Autodesk Inventor part; units mm, degrees
ref_plane "YZ Plane" through (0, 0, 0) normal (1, 0, 0) x (0, 1, 0)
ref_plane "XZ Plane" through (0, 0, 0) normal (0, 1, 0) x (-1, 0, 0)
ref_plane "XY Plane" through (0, 0, 0) normal (0, 0, 1) x (1, 0, 0)
sketch "Sketch1" plane through (0, 0, 0) normal (0, 0, 1) x (1, 0, 0)
  line L0 (0, 0) -> (88.9, 0)
  line L1 (88.9, 0) -> (88.9, 12.7)
  line L2 (0, 12.7) -> (0, 0)
  line L3 (0, 12.7) -> (0, 0)
  circle A0 centre (37.338, 50.8) radius 14.2875
  line L4 (0, 0) -> (0, 12.7)
  line L5 (0, 0) -> (0, 12.7)
  line L6 (0, 12.7) -> (15.748, 12.7)
  line L7 (13.208, 0) -> (0, 0)
  line L8 (15.748, 12.7) -> (0, 12.7)
  line L9 (15.748, 54.61) -> (15.748, 12.7)
  line L10 (88.9, 0) -> (62.992, 0)
  line L11 (73.152, 12.7) -> (88.9, 12.7)
  line L12 (88.9, 12.7) -> (88.9, 0)
  line L13 (73.152, 12.7) -> (73.152, 54.61)
  line L14 (60.452, 71.222) -> (28.448, 71.222)
  line L15 (15.748, 54.61) -> (15.748, 58.522)
  line L16 (73.152, 58.522) -> (73.152, 54.61)
  arc A1 (28.448, 71.222) -> (15.748, 58.522) centre (28.448, 58.522) ccw
  arc A2 (73.152, 58.522) -> (60.452, 71.222) centre (60.452, 58.522) ccw
  point P0 (65.9232, 76.2)
  point P1 (0, 12.7)
  dimension "d9" = 28.575
  dimension "d10" = 88.9
  dimension "d56" = 12.7
  dimension "d57" = 15.748
  dimension "d79" = 21.59
  dimension "d83" = 15.748
  dimension "d87" = 12.7
  dimension "d111" = 41.91
  dimension "d112" = 41.91
  dimension "d118" = 25.4
  dimension "d119" = 12.7
extrude "Extrusion7" add sketch "Sketch1" along normal blind 15.24
sketch "Sketch9" plane through (73.152, 12.7, 0) normal (0, 1, 0) x (1, 0, 0)
  point P0 (-73.152, 0)
  point P1 (8.0463, -7.7031)
hole "Hole4" at (81.1983, 12.7, 7.7031) direction (0, -1, 0) diameter 6.4008 end through all counterbore diameter 11.9062 counterbore depth 7.9502
sketch "Sketch10" plane through (0.0713, 12.7, -0.0767) normal (0, 1, 0) x (1, 0, 0)
  point P0 (-75.692, 0)
  point P1 (7.4278, -7.7745)
hole "Hole5" at (7.4991, 12.7, 7.6977) direction (0, -1, 0) diameter 6.4008 end through all counterbore diameter 11.9062 counterbore depth 7.9502
properties part number "Updated Support_chris"
The listing builds one solid part. Answer for the finished solid, in the listing's coordinates (mm). A direction names the side the tool comes from. Give positions to 0.01 mm unless a question says otherwise; leave off trailing zeros. Order: outer loops, then holes, each group sorted by start corner. A loop starts at its lowest first (then second) coordinate and runs counter-clockwise, first axis right, second up. Notation, with made-up numbers: M 61.25,-12 L 119.25,-12 A20 cw 119.25,17 Z; hole C -11.75,-9 d7. An arc over 180 degrees is marked long. Put each result on its own line as item: value. Start each with the question number.
Item 1: The part is cut by section C-C, the plane x = 12. Determine the outline of the cut face in (y, z), and give its area (3 significant figures).
Item 2: For a pull along Z with two mould halves and no side action, classify faces 1 (the face through (44, 28, 15.24)), 2 (the face through (45, 71.222, 8)), 3 (the face through (80.237, 2.342, 10.756)), 4 (the face through (4.326, 2.342, 7.281)) as +Z half, -Z half, draft (parallel to the pull), parting line (faces both ways), or undercut.
Item 3: The part is cut by section D-D, the plane y = 15.5. Determine the outline of the cut face in (x, z), and give its area (3 significant figures).
Item 4: Flat-ended cylindrical pins translate along their axes: P1, Ø1, axis at x = 67.5, z = 3.5, coming from the -Y side; P2, Ø17, axis at x = 37.338, y = 50.8, coming from the -Z side (3 decimals); P3, Ø2, axis at y = 60, z = 9.5, coming from the -X side; P4, Ø1, axis at y = 36.5, z = 2, coming from the -X side. Find the tip coordinate at first contact, or state that the pin passes through.
Item 5: The part is cut by section B-B, the plane y = 50.8. Determine the outline of the cut face in (x, z), and give its area (3 significant figures).
Item 6: The part is cut by section A-A, the plane z = 8. Determine the outline of the cut face in (x, y) (1 decimal), and give its area (3 significant figures).
Item 7: Find the intervals of material crossed by line 1 along X through (y, z) = (16, 7.75); line 2 along X through (y, z) = (48.5, 7.5); line 3 along Y through (x, z) = (76, 1.25), in increasing order.
Item 8: Which of the six approach directions +Z, -Z, +X, -X, +Y, -Y give full straight-line access (tool end or side, diameter ignored) to faces 5 (the face through (77, 12.7, 2)), 6 (the face through (10, 4.75, 10)), 7 (the face through (15.748, 36, 8))?
Answer key:
1. outline: M 0,0 L 12.7,0 L 12.7,3.8 L 4.75,3.8 L 4.75,11.59 L 12.7,11.59 L 12.7,15.24 L 0,15.24 Z
1. area: 132 mm²
2. face 1: +Z half
2. face 2: draft
2. face 3: undercut
2. face 4: undercut
3. outline: M 15.75,0 L 73.15,0 L 73.15,15.24 L 15.75,15.24 Z
3. area: 875 mm²
4. P1: stops at y = 0
4. P2: passes through
4. P3: stops at x = 15.76
4. P4: stops at x = 15.75
5. outline: M 15.75,0 L 23.05,0 L 23.05,15.24 L 15.75,15.24 Z; M 51.63,0 L 73.15,0 L 73.15,15.24 L 51.63,15.24 Z
5. area: 439 mm²
6. outline: M 0,0 L 4.3,0 L 4.3,4.7 L 1.6,4.7 L 1.6,12.7 L 0,12.7 Z; M 10.7,0 L 78,0 L 78,4.7 L 75.3,4.7 L 75.3,12.7 L 73.2,12.7 L 73.2,58.5 A12.7 ccw 60.5,71.2 L 28.4,71.2 A12.7 ccw 15.7,58.5 L 15.7,12.7 L 13.4,12.7 L 13.4,4.7 L 10.7,4.7 Z; M 84.4,0 L 88.9,0 L 88.9,12.7 L 87.1,12.7 L 87.1,4.7 L 84.4,4.7 Z; hole C 37.3,50.8 d28.6
6. area: 3,530 mm²
7. line 1: x = 15.75 to 73.15
7. line 2: x = 15.75 to 23.24, 51.44 to 73.15
7. line 3: y = 0 to 12.7
8. face 5: +Z, -Z, +X, +Y
8. face 6: +Y
8. face 7: +Z, -Z, -X, +Y
